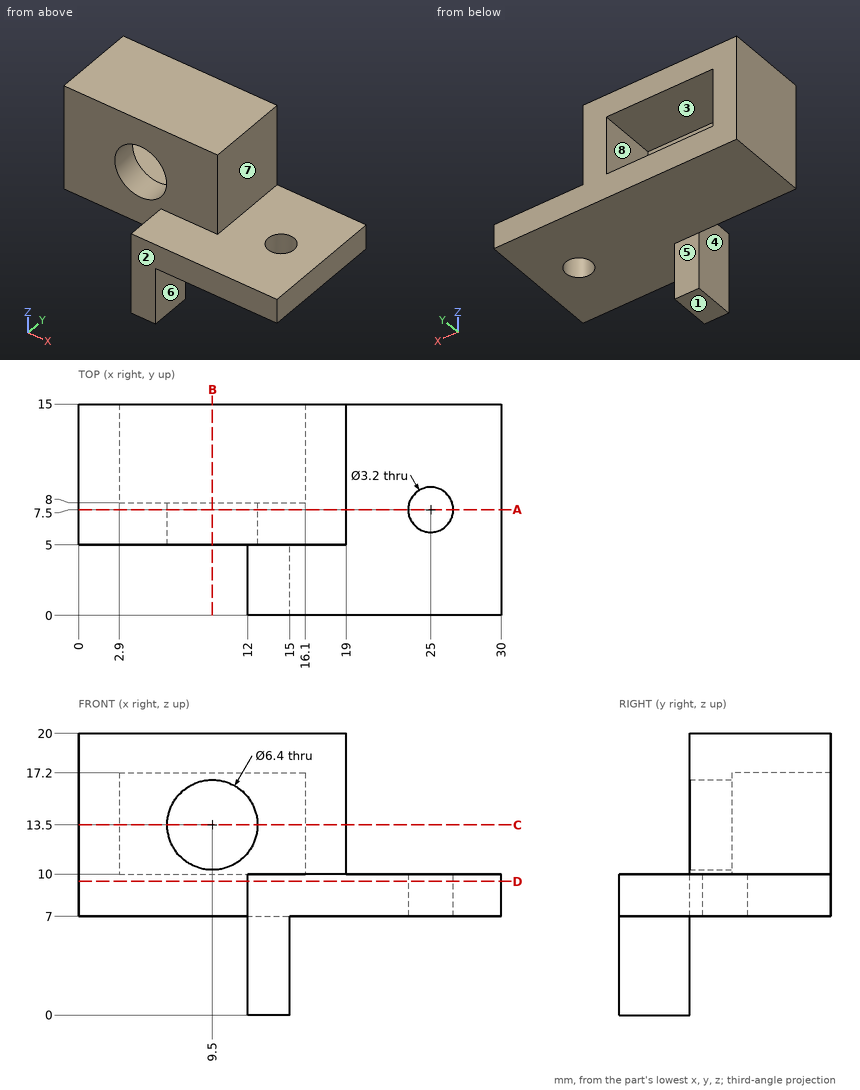
The drawing under review shows one solid part. Ordinate dimensions are in mm from its lowest x, y, z. A direction names the side the tool comes from. Coordinates: 2 decimals unless noted, no trailing zeros. Loops run counter-clockwise (first coordinate to the right, second up) from the corner with the lowest first, then second, coordinate; pieces in that order, holes last. Notation, with made-up numbers: (-38, 85.5) -> (6, 85.5) arc R23 ccw to (6, 102.5) -> close; hole circle Ø8 at (-4, -8.5). An arc over 180 degrees is marked (long way). Answer as a JSON object with one key per item and string values.
Q1. Take a section at D-D on z = 9.5. Give the boundary of the cut face in (x, y), plus the area to 3 significant figures.
Answer block:
{"outline": "(0, 5) -> (12, 5) -> (12, 0) -> (30, 0) -> (30, 15) -> (0, 15) -> close; hole circle Ø3.2 at (25, 7.5)", "area": "382 mm^2"}
Q2. To check wall thickness, follow L1, parallel to Z at x = 9.5, y = 6.7; L2, parallel to X at y = 6.25, z = 13.5; L3, parallel to X at y = 9.75, z = 16.5. State the ranges of each line that lie inside material, in increasing order.
Answer block:
{"L1": "z = 7 to 10.3, 16.7 to 20", "L2": "x = 0 to 6.3, 12.7 to 19", "L3": "x = 0 to 2.9, 16.1 to 19"}
Q3. Take a section at B-B on x = 9.5. Give the boundary of the cut face in (y, z), plus the area to 3 significant figures.
Answer block:
{"outline": "(5, 7) -> (15, 7) -> (15, 10) -> (8, 10) -> (8, 10.3) -> (5, 10.3) -> close; (5, 16.7) -> (8, 16.7) -> (8, 17.2) -> (15, 17.2) -> (15, 20) -> (5, 20) -> close", "area": "60.4 mm^2"}
Q4. Take a section at A-A on y = 7.5. Give the boundary of the cut face in (x, z), plus the area to 3 significant figures.
Answer block:
{"outline": "(0, 7) -> (23.4, 7) -> (23.4, 10) -> (19, 10) -> (19, 20) -> (0, 20) -> close; (26.6, 7) -> (30, 7) -> (30, 10) -> (26.6, 10) -> close; hole circle Ø6.4 at (9.5, 13.5)", "area": "238 mm^2"}
Q5. Tool access review of the marked faces 4, 5, 6, 7 and 8: name each direction out of +Z, -Z, +X, -X, +Y, -Y from which nothing blocks a thin tool from reaching the whole face with its end or side.
Answer block:
{"face 4": "+Z, -Z, -X, -Y", "face 5": "-Z, +X, -X, +Y", "face 6": "-Z, +X, +Y, -Y", "face 7": "+Z, +X, +Y, -Y", "face 8": "+Y"}
Q6. The part is to be moulded in two halves that separate along Z. For the marked faces 1, 2 and 3, say which applies: +Z half, -Z half, draft (parallel to the pull), parting line (faces both ways), or undercut.
Answer block:
{"face 1": "-Z half", "face 2": "draft", "face 3": "undercut"}
Q7. Clearance check with flat-ended pins moving along their axes: pin 1 Ø4.5 at (x, y) = (17, 9) entering from -Z; pin 2 Ø8 at (x, z) = (12, 14) entering from +Y; pin 3 Ø7.5 at (x, y) = (23, 4.5) entering from +Z; pin 4 Ø2 at (y, z) = (13, 12) entering from +X. State where each tip first meets the part, or that it passes through.
Answer block:
{"pin 1": "stops at z = 7", "pin 2": "stops at y = 15", "pin 3": "stops at z = 10", "pin 4": "stops at x = 19"}
Q8. Take a section at C-C on z = 13.5. Give the boundary of the cut face in (x, y), plus the area to 3 significant figures.
Answer block:
{"outline": "(0, 5) -> (6.3, 5) -> (6.3, 8) -> (2.9, 8) -> (2.9, 15) -> (0, 15) -> close; (12.7, 5) -> (19, 5) -> (19, 15) -> (16.1, 15) -> (16.1, 8) -> (12.7, 8) -> close", "area": "78.4 mm^2"}
